Read the model definition and answer for the solid it produces. Units are mm, in the model's axes. Face numbers are marked on the shaded views. A direction names the side the tool comes from. Round coordinates to 2 decimals unless told otherwise and drop trailing zeros. Write each loop counter-clockwise with the first axis right and the second up, starting at its lowest first coordinate (ties: lowest second). Pieces come first, ordered by that corner, then holes. Notation, with made-up numbers: (48.25, 80.25) -> (86.25, 80.25) arc R34 cw to (86.25, 114.25) -> close; hole circle Ø10 at (42, 38). An arc over 180 degrees is marked (long way). Return JSON: item names as keys, results as strings.
Autodesk Inventor part; units mm, degrees
ref_plane "Work Plane1" through (22, 0, 0) normal (1, 0, 0) x (0, 0, -1)
ref_plane "Work Plane2" through (0, 5, 0) normal (0, 1, 0) x (-1, 0, 0)
ref_plane "YZ Plane" through (0, 0, 0) normal (1, 0, 0) x (0, 1, 0)
sketch "Sketch1" plane through (0, 0, 0) normal (1, 0, 0) x (0, 1, 0)
  circle A0 centre (0, 0) radius 2.25
  dimension "diameter" = 4.5
extrude "Extrusion1" add sketch "Sketch1" along normal blind 20
ref_plane "Work Plane1" through (22, 0, 0) normal (1, 0, 0) x (0, 0, -1)
sketch "Sketch3" plane through (22, 0, 0) normal (1, 0, 0) x (0, 0, -1)
  arc A0 (-1.75, 1.7854) -> (-1.75, -1.7854) centre (0, 0) ccw construction
  line L0 (-1.75, -1.7854) -> (1.75, -1.7854) construction
  line L1 (1.75, -1.7854) -> (1.75, 1.7854)
  line L2 (1.75, 1.7854) -> (-1.75, 1.7854) construction
  line L3 (-1.75, 1.7854) -> (-1.75, -1.7854)
  line L4 (-1.75, -1.7854) -> (1.75, 1.7854) construction
  line L5 (1.75, -1.7854) -> (0, 0) construction
  arc A1 (1.75, 1.7854) -> (-1.75, 1.7854) centre (0, 0) ccw
  arc A2 (1.75, -1.7854) -> (1.75, 1.7854) centre (0, 0) ccw construction
  arc A3 (-1.75, -1.7854) -> (1.75, -1.7854) centre (0, 0) ccw
  line L6 (0, 0) -> (-1.75, 1.7854) construction
  dimension "d23" = 5
  dimension "d34" = 3.5
extrude "Extrusion3" add sketch "Sketch3" along normal blind 5
loft "Loft1" add section 1 edges at (22, 2.5, 0) (22, 0, -1.75) (22, -2.5, 0) (22, 0, 1.75) section 2 edges at (20, -2.25, 0)
sketch "Sketch4" plane through (27, 0, 0) normal (1, 0, 0) x (0, 0, -1)
  arc A0 (1.75, 1.7854) -> (-1.75, 1.7854) centre (0, 0) ccw
hole "Hole1" at (27, 0, 0) direction (-1, 0, 0) diameter 2 depth 6
mirror "Mirror1" about plane through (0, 0, 0) normal (-1, 0, 0)
ref_plane "Work Plane2" through (0, 5, 0) normal (0, 1, 0) x (-1, 0, 0)
sketch "Sketch5" plane through (0, 5, 0) normal (0, 1, 0) x (-1, 0, 0)
  point P0 (0, 0)
  point P1 (0, 0)
hole "Hole2" at (0, 5, 0) direction (0, -1, 0) diameter 3 end through all counterbore diameter 6 counterbore depth 2
properties part number "front shaft v2"
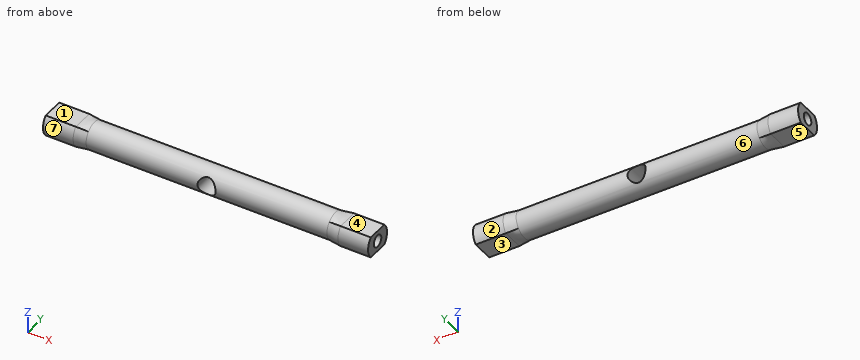
Item 1: For a pull along X with two mould halves and no side action, classify the marked faces 6 and 7 as released by +X, released by -X, zero draft, split by the parting line, or undercut.
Worked answers:
{"face 6": "undercut", "face 7": "zero draft"}
Item 2: A tool of negligible diameter and unlimited length cuts with its end or side. For the marked faces 1, 2, 3, 4 and 5, from which of +Z, -Z, +X, -X, +Y, -Y can it reach the whole face along a straight path? Write none if from no direction.
Worked answers:
{"face 1": "+Z, -X, +Y, -Y", "face 2": "+X, -X, +Y", "face 3": "-Z, +X, +Y, -Y", "face 4": "+Z, +X, +Y, -Y", "face 5": "-Z, -X, +Y, -Y"}
Item 3: Section C-C (x = 17) is taken. Give the vertices of the cut face in (y, z), then the cut area to 3 significant figures.
Worked answers:
{"outline": "circle Ø4.5 at (0, 0)", "area": "15.9 mm2"}
Item 4: Section B-B (x = 0) is taken. Give the vertices of the cut face in (y, z), then the cut area to 3 significant figures.
Worked answers:
{"outline": "(-1.68, -1.5) arc R2.25 ccw to (1.68, -1.5) -> close; (-1.68, 1.5) -> (1.68, 1.5) arc R2.25 ccw to start", "area": "3.48 mm2"}
Item 5: Straight lines are drawn through the part: L1, parallel to Y at x = 22.4, z = 0; L2, parallel to Z at x = -23.2, y = 0; L3, parallel to X at y = -1.1, z = 0. For each, find the intervals that lie inside material, in ascending order. Write a range as [from, to].
Worked answers:
{"L1": "y = [-2.5, -1], [1, 2.5]", "L2": "z = [-1.75, -1], [1, 1.75]", "L3": "x = [-27, -1.5], [1.5, 27]"}
Item 6: Flat-ended cylindrical pins translate along their axes: pin 1 (1.6 mm diameter, centred on y = 0, z = 0, fed in from -X); pin 2 (1.5 mm diameter, centred on x = 20, z = -1, fed in from -Y); pin 3 (1.8 mm diameter, centred on x = -24, y = 0.5, fed in from +Z). Find the tip coordinate at first contact, or state that the pin passes through.
Worked answers:
{"pin 1": "stops at x = -21", "pin 2": "stops at y = -2.27", "pin 3": "stops at z = 1.75"}
Item 7: Section A-A (z = 0) is taken. Give the vertices of the cut face in (x, y).
Worked answers:
{"outline": "(-27, -2.5) -> (-22, -2.5) -> (-20, -2.25) -> (-1.5, -2.25) -> (-1.5, 2.25) -> (-20, 2.25) -> (-22, 2.5) -> (-27, 2.5) -> (-27, 1) -> (-21, 1) -> (-21, -1) -> (-27, -1) -> close; (1.5, -2.25) -> (20, -2.25) -> (22, -2.5) -> (27, -2.5) -> (27, -1) -> (21, -1) -> (21, 1) -> (27, 1) -> (27, 2.5) -> (22, 2.5) -> (20, 2.25) -> (1.5, 2.25) -> close"}
